Geometry check sheet. Reference: the model listing, model coordinates, mm. Give positions to 0.01 mm unless a question says otherwise; leave off trailing zeros. Order: outer loops, then holes, each group sorted by start corner. A loop starts at its lowest first (then second) coordinate and runs counter-clockwise, first axis right, second up.
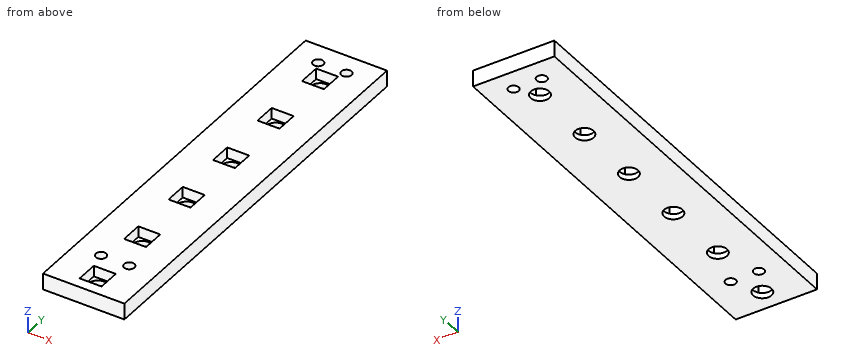
Autodesk Fusion 360 part; units mm, degrees
sketch "Schizzo1" plane through (0, 0, 0) normal (0, 0, 1) x (1, 0, 0)
  line L0 (25.7791, 75.2827) -> (55.7791, 75.2827)
  line L1 (55.7791, 75.2827) -> (55.7791, -74.7173)
  line L2 (55.7791, -74.7173) -> (25.7791, -74.7173)
  line L3 (25.7791, -74.7173) -> (25.7791, 75.2827)
  line L4 (40.7791, 75.2827) -> (40.7791, -74.7173) construction
  line L5 (25.7791, 0.2827) -> (55.7791, 0.2827) construction
  circle A0 centre (40.7791, 60.2827) radius 3.4
  line L6 (44.8291, 56.2327) -> (36.7291, 56.2327)
  line L7 (36.7291, 56.2327) -> (36.7291, 64.3327)
  line L8 (36.7291, 64.3327) -> (44.8291, 64.3327)
  line L9 (44.8291, 64.3327) -> (44.8291, 56.2327)
  line L10 (44.8291, 56.2327) -> (36.7291, 64.3327) construction
  line L11 (36.7291, 56.2327) -> (44.8291, 64.3327) construction
  line L12 (44.8291, 38.9327) -> (44.8291, 30.8327)
  line L13 (36.7291, 38.9327) -> (44.8291, 38.9327)
  line L14 (36.7291, 30.8327) -> (36.7291, 38.9327)
  circle A1 centre (40.7791, 34.8827) radius 3.4
  line L15 (44.8291, 30.8327) -> (36.7291, 30.8327)
  line L16 (44.8291, 13.5327) -> (44.8291, 5.4327)
  line L17 (36.7291, 13.5327) -> (44.8291, 13.5327)
  line L18 (36.7291, 5.4327) -> (36.7291, 13.5327)
  circle A2 centre (40.7791, 9.4827) radius 3.4
  line L19 (44.8291, 5.4327) -> (36.7291, 5.4327)
  line L20 (44.8291, -11.8673) -> (44.8291, -19.9673)
  line L21 (36.7291, -11.8673) -> (44.8291, -11.8673)
  line L22 (36.7291, -19.9673) -> (36.7291, -11.8673)
  circle A3 centre (40.7791, -15.9173) radius 3.4
  line L23 (44.8291, -19.9673) -> (36.7291, -19.9673)
  line L24 (44.8291, -37.2673) -> (44.8291, -45.3673)
  line L25 (36.7291, -37.2673) -> (44.8291, -37.2673)
  line L26 (36.7291, -45.3673) -> (36.7291, -37.2673)
  circle A4 centre (40.7791, -41.3173) radius 3.4
  line L27 (44.8291, -45.3673) -> (36.7291, -45.3673)
  line L28 (44.8291, -62.6673) -> (44.8291, -70.7673)
  line L29 (36.7291, -62.6673) -> (44.8291, -62.6673)
  line L30 (36.7291, -70.7673) -> (36.7291, -62.6673)
  circle A5 centre (40.7791, -66.7173) radius 3.4
  line L31 (44.8291, -70.7673) -> (36.7291, -70.7673)
  line L32 (35.5791, 75.2827) -> (35.5791, -74.7173) construction
  circle A6 centre (35.5791, 67.2827) radius 1.9
  circle A7 centre (45.9791, 67.2827) radius 1.9
  circle A8 centre (35.5791, -56.7173) radius 1.9
  circle A9 centre (45.9791, -56.7173) radius 1.9
  point P0 (40.7791, 60.2827)
  dimension "d1" = 30
  dimension "d2" = 150
  dimension "d3" = 6.8
  dimension "d4" = 8.1
  dimension "d5" = 8.1
  dimension "d8" = 25.4
  dimension "d9" = 0
  dimension "d11" = 15
  dimension "d22" = 5.2
  dimension "d23" = 3.8
  dimension "d24" = 8
  dimension "d27" = 124
  dimension "d28" = 0
  dimension "d29" = 25.4
  dimension "d30" = 124
extrude "Estrusione1" add sketch "Schizzo1" along normal blind 6 contours L0 L1 L2 L3
extrude "Estrusione2" add sketch "Schizzo1" along normal blind 2 contours L6 L7 L8 L9 | L12 L13 L14 L15 | L16 L17 L18 L19 | L20 L21 L22 L23 | L24 L25 L26 L27 | L28 L29 L30 L31
Q1. Thickness scan on L1, parallel to X at y = -67.5, z = 0.4; L2, parallel to Y at x = 35.5, z = 0.6; L3, parallel to Y at x = 45.5, z = 1.45. Record the ranges inside material, lowest first.
Q2. Cross-section at A-A, the plane z = 0.9. Give the number of separate pieces and of enclosed holes in the cut face, and give its area (3 significant figures).
Q3. Gauge pin test, flat end, axial feed: P1, Ø2.5, axis at x = 39, y = 33, coming from the +Z side. Record the tip position at first contact, or that the pin passes through.
Q4. Cross-section at B-B, the plane x = 46.5. Record the boundary of the cut face in (y, z).
Answers follow:
1. L1: x = 25.78 to 37.47, 44.09 to 55.78
1. L2: y = -74.72 to -58.62, -54.82 to 65.38, 69.18 to 75.28
1. L3: y = -74.72 to -58.56, -54.88 to 65.44, 69.12 to 75.28
2. separate pieces: 1
2. enclosed holes: 10
2. area: 4,240 mm2
3. P1: stops at z = 2
4. outline: (-74.72, 0) - (-58.54, 0) - (-58.54, 6) - (-74.72, 6) - close; (-54.89, 0) - (65.46, 0) - (65.46, 6) - (-54.89, 6) - close; (69.11, 0) - (75.28, 0) - (75.28, 6) - (69.11, 6) - close
